Geometry: see drawing. Coordinates: mm, zero at the bounding-box minimum. A direction names the side the tool comes from. Give positions to 0.01 mm unless a question says otherwise; leave off trailing zeros. Write each loop counter-clockwise with the first axis right and the second up, starting at its lowest first coordinate (ties: lowest second). Pieces come first, ordered by that corner, then holes. Notation, with made-up numbers: (20, 84.5) -> (74, 84.5) arc R29 ccw to (74, 107.5) -> close; hole circle Ø6 at (76, 42). An arc over 180 degrees is marked (long way). Write item = value, one per line.
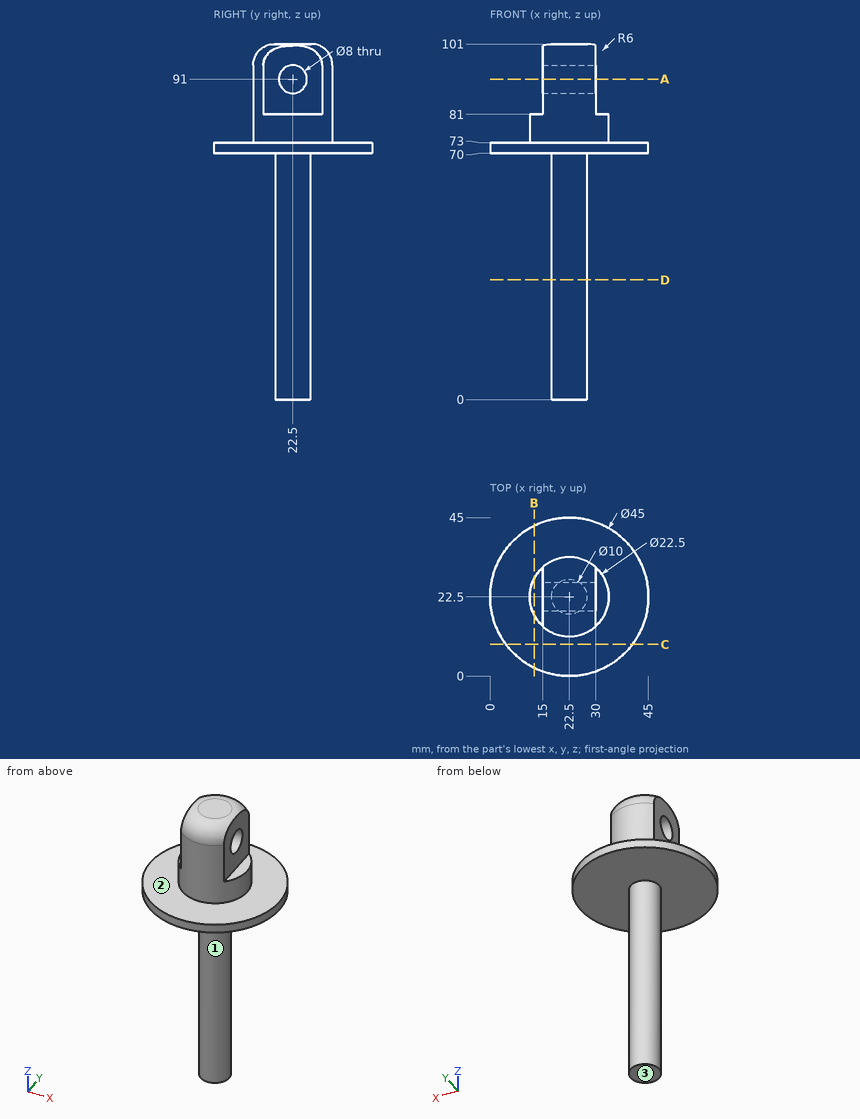
(1) Material intervals for line 1 (Z direction, x = 22.5, y = 22.5); line 2 (Y direction, x = 23, z = 76); line 3 (Z direction, x = 7.5, y = 8.5), sorted ascending.
Values follow:
line_1 = 0 to 87, 95 to 101
line_2 = 11.26 to 33.74
line_3 = 70 to 73
(2) Section query A-A (z = 91). Return loops of the section in (x, y).
Values follow:
outline = (15, 14.11) arc R11.25 ccw to (30, 14.11) -> (30, 18.5) -> (15, 18.5) -> close; (15, 26.5) -> (30, 26.5) -> (30, 30.89) arc R11.25 ccw to (15, 30.89) -> close
(3) Section query D-D (z = 34). Return loops of the section in (x, y).
Values follow:
outline = circle Ø10 at (22.5, 22.5)
(4) First-contact query: pin 1 (1.1 mm diameter, centred on x = 31, y = 22.5, fed in from +Z); pin 2 (12 mm diameter, centred on y = 40, z = 64.5, fed in from +X); pin 3 (12 mm diameter, centred on y = 15, z = 78, fed in from -X). Flat tips, straight axial feed; report the tip coordinate or a pass-through.
Values follow:
pin_1 = 81
pin_2 = 39.18
pin_3 = 0.39
(5) Access query for the marked faces 1, 2 and 3. Directions: +Z, -Z, +X, -X, +Y, -Y. A direction counts if a zero-diameter tool reaches every point of the face in a straight line with its end or side. Return the directions, or none.
Values follow:
face_1 = -Z
face_2 = +Z
face_3 = -Z, +X, -X, +Y, -Y
(6) Section query B-B (x = 12.5). Return loops of the section in (y, z).
Values follow:
outline = (2.34, 70) -> (42.66, 70) -> (42.66, 73) -> (27.65, 73) -> (27.65, 81) -> (17.35, 81) -> (17.35, 73) -> (2.34, 73) -> close
(7) Section query C-C (y = 9). Return loops of the section in (x, z), plus the area to 3 significant figures.
Values follow:
outline = (4.5, 70) -> (40.5, 70) -> (40.5, 73) -> (4.5, 73) -> close
area = 108 mm2
